CAD build for the part. Positions are in the model's coordinates, mm. Round coordinates to 2 decimals unless told otherwise and drop trailing zeros. Loops run counter-clockwise (first coordinate to the right, second up) from the corner with the lowest first, then second, coordinate; pieces in that order, holes last.
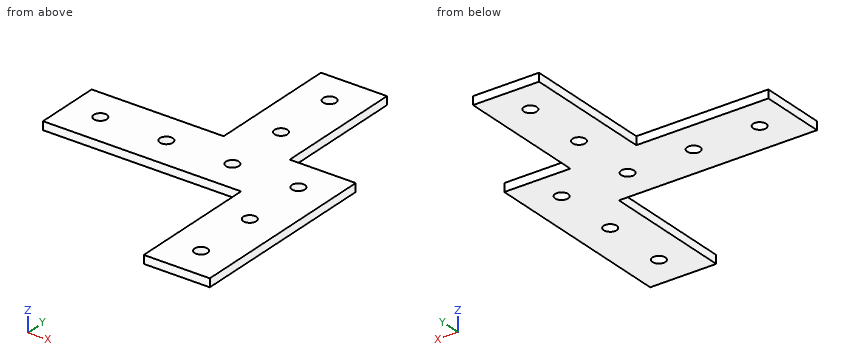
```python
from build123d import *

# Parameters (mm, degrees)
F0_R     = 2.4892
F1_DEPTH = 3.175


with BuildPart() as f1:
    # F0 (on Top) → F1 (new body)
    with BuildSketch(Plane.XY):
        Polygon((-88.9, 63.5), (-88.9, 38.1), (-12.7, 38.1), (-12.7, -12.7), (12.7, -12.7), (12.7, 63.5), (-12.7, 63.5), (-12.7, 114.3), (-38.1, 114.3), (-38.1, 63.5), align=None)
        Circle(F0_R, mode=Mode.SUBTRACT)
        with Locations((0, 25.4)):
            Circle(F0_R, mode=Mode.SUBTRACT)
        with Locations((-76.2, 50.8)):
            Circle(F0_R, mode=Mode.SUBTRACT)
        with Locations((-50.8, 50.8)):
            Circle(F0_R, mode=Mode.SUBTRACT)
        with Locations((-25.4, 50.8)):
            Circle(F0_R, mode=Mode.SUBTRACT)
        with Locations((-25.4, 76.2)):
            Circle(F0_R, mode=Mode.SUBTRACT)
        with Locations((0, 50.8)):
            Circle(F0_R, mode=Mode.SUBTRACT)
        with Locations((-25.4, 101.6)):
            Circle(F0_R, mode=Mode.SUBTRACT)
    extrude(amount=F1_DEPTH)


solid = f1.part
```
Item 1: Probe line 1 (Y direction, x = -76.2, z = 2.3); line 2 (Y direction, x = -60.5, z = 3); line 3 (X direction, y = 88, z = 0.5). List the from-to ranges inside material, lowest first.
Answers follow:
line 1: y = 38.1 to 48.31, 53.29 to 63.5
line 2: y = 38.1 to 63.5
line 3: x = -38.1 to -12.7
Item 2: Cut at D-D, the plane x = -51.5. Give the cut face in (y, z) (3 decimals).
Answers follow:
outline: (38.1, 0) - (48.411, 0) - (48.411, 3.175) - (38.1, 3.175) - close; (53.189, 0) - (63.5, 0) - (63.5, 3.175) - (53.189, 3.175) - close
Item 3: Flat gauge pins, fed straight in: P1, Ø5.5, axis at x = -25.4, y = 50.8, coming from the -Z side; P2, Ø1, axis at y = 24, z = 2.5, coming from the -X side; P3, Ø1.6, axis at y = 99.5, z = 2, coming from the -X side; P4, Ø1.5, axis at x = -71, z = 2, coming from the -Y side. Where does each tip first touch, or does it go through?
Answers follow:
P1: stops at z = 0
P2: stops at x = -12.7
P3: stops at x = -38.1
P4: stops at y = 38.1
Item 4: Cut at B-B, the plane x = 0. Give the cut face in (y, z) (3 decimals).
Answers follow:
outline: (-12.7, 0) - (-2.489, 0) - (-2.489, 3.175) - (-12.7, 3.175) - close; (2.489, 0) - (22.911, 0) - (22.911, 3.175) - (2.489, 3.175) - close; (27.889, 0) - (48.311, 0) - (48.311, 3.175) - (27.889, 3.175) - close; (53.289, 0) - (63.5, 0) - (63.5, 3.175) - (53.289, 3.175) - close
Item 5: Cut at A-A, the plane y = 25.4. Give the cut face in (x, z) (3 decimals), plus the area to 3 significant figures.
Answers follow:
outline: (-12.7, 0) - (-2.489, 0) - (-2.489, 3.175) - (-12.7, 3.175) - close; (2.489, 0) - (12.7, 0) - (12.7, 3.175) - (2.489, 3.175) - close
area: 64.8 mm2
Item 6: Cut at C-C, the plane z = 0.8. State how many separate pieces and enclosed holes the cut face has, plus the area to 3 significant figures.
Answers follow:
separate pieces: 1
enclosed holes: 8
area: 5,010 mm2
